```python
from build123d import *

# Parameters (mm, degrees)
F0_R     = 12.7
F1_DEPTH = 76.2
F4_W     = 3.175
F4_H     = 12.7
F5_DEPTH = 12.7
F6_R     = 1.27
F7_DEPTH = 12.7


with BuildPart() as f1:
    # F0 (on Top) → F1 (new body)
    with BuildSketch(Plane.XY):
        Circle(F0_R)
    extrude(amount=F1_DEPTH)

    # F2 (on Front) → F3 (revolve, cut)
    with BuildSketch(Plane.XZ):
        Polygon((-17.214077, -2.216983), (-3.175, 4.865219), (-3.175, 83.753079), (-17.214077, 83.753079), align=None)
    revolve(axis=Axis((0, 0, 76.2), (0, 0, 1)), mode=Mode.SUBTRACT)

    # F4 (on Front) → F5 (cut, symmetric)
    with BuildSketch(Plane.XZ):
        with Locations((0, 76.409727)):
            Rectangle(F4_W, F4_H)
    extrude(amount=F5_DEPTH, both=True, mode=Mode.SUBTRACT)

    # F6 (on Right) → F7 (cut, symmetric)
    with BuildSketch(Plane.YZ):
        with Locations((0, 74.752115)):
            Circle(F6_R)
    extrude(amount=F7_DEPTH, both=True, mode=Mode.SUBTRACT)


solid = f1.part
```
Geometry check sheet. Reference: the model listing, model coordinates, mm. A direction names the side the tool comes from. Round coordinates to 2 decimals unless told otherwise and drop trailing zeros. Loops run counter-clockwise (first coordinate to the right, second up) from the corner with the lowest first, then second, coordinate; pieces in that order, holes last. Notation, with made-up numbers: (40.5, 64) - (93.5, 64) arc R18 cw to (93.5, 96) - close; hole circle Ø4 at (1, 3.5). An arc over 180 degrees is marked (long way). Write each question's results on one line, items separated by ' | '. Start each with the question number.
Q1. Access from +Z, -Z, +X, -X, +Y, -Y to the whole of each face (thin tool, end or side, straight path). Record for faces 4 (the flat face through (0, 0, 70.06)), 5 (the cylindrical face through (0.41, -3.15, 41.03)), 6 (the flat face through (2, 0, 76.2)).
Q2. Gauge pin test, flat ends, axial feed: P1, Ø6, axis at y = -3.5, z = 44, coming from the +X side; P2, Ø2.5, axis at x = -0.5, y = 1.5, coming from the +Z side; P3, Ø2.5, axis at y = -0.5, z = 72, coming from the +X side (3 decimals); P4, Ø6, axis at y = 1, z = 72, coming from the -X side (3 decimals). Record the tip position at first contact, or that the pin passes through.
Q3. Thickness scan on line 1 (Z direction, x = 2.5, y = 0); line 2 (X direction, y = 0.25, z = 58); line 3 (X direction, y = 2, z = 71). Record the ranges inside material, lowest first. Write a range as [from, to].
Q4. Cross-section at D-D on z = 38.5. Enter the section's corners in (x, y) (3 decimals).
Q5. Cross-section at A-A on y = 0. State how many separate pieces and enclosed holes the cut face has, and give its area (3 significant figures).
Q6. Release check for a two-part mould opening along X. For faces 1 (the flat face through (-2, 0, 76.2)), 2 (the flat face through (-1.588, 0, 72)), 3 (the conical face through (0.79, 3.55, 4.63)) record: +X half, -X half, draft (parallel to the pull), parting line (faces both ways), or undercut.
Q7. Cross-section at C-C on x = 0. Enter the section's corners in (y, z) (3 decimals).
Answers below:
1) face 4: +Z, +Y, -Y | face 5: +Z | face 6: +Z, +X, -X, +Y, -Y
2) P1: stops at x = 3.14 | P2: stops at z = 76.2 | P3: stops at x = 3.175 | P4: stops at x = -3.175
3) line 1: z = [0, 73.48], [76.02, 76.2] | line 2: x = [-3.17, 3.17] | line 3: x = [-2.47, -1.59], [1.59, 2.47]
4) outline: circle Ø6.35 at (0, 0)
5) separate pieces: 3 | enclosed holes: 0 | area: 503 mm²
6) face 1: draft | face 2: undercut | face 3: parting line
7) outline: (-12.7, 0) - (12.7, 0) - (12.7, 0.06) - (3.175, 4.865) - (3.175, 70.06) - (-3.175, 70.06) - (-3.175, 4.865) - (-12.7, 0.06) - close
